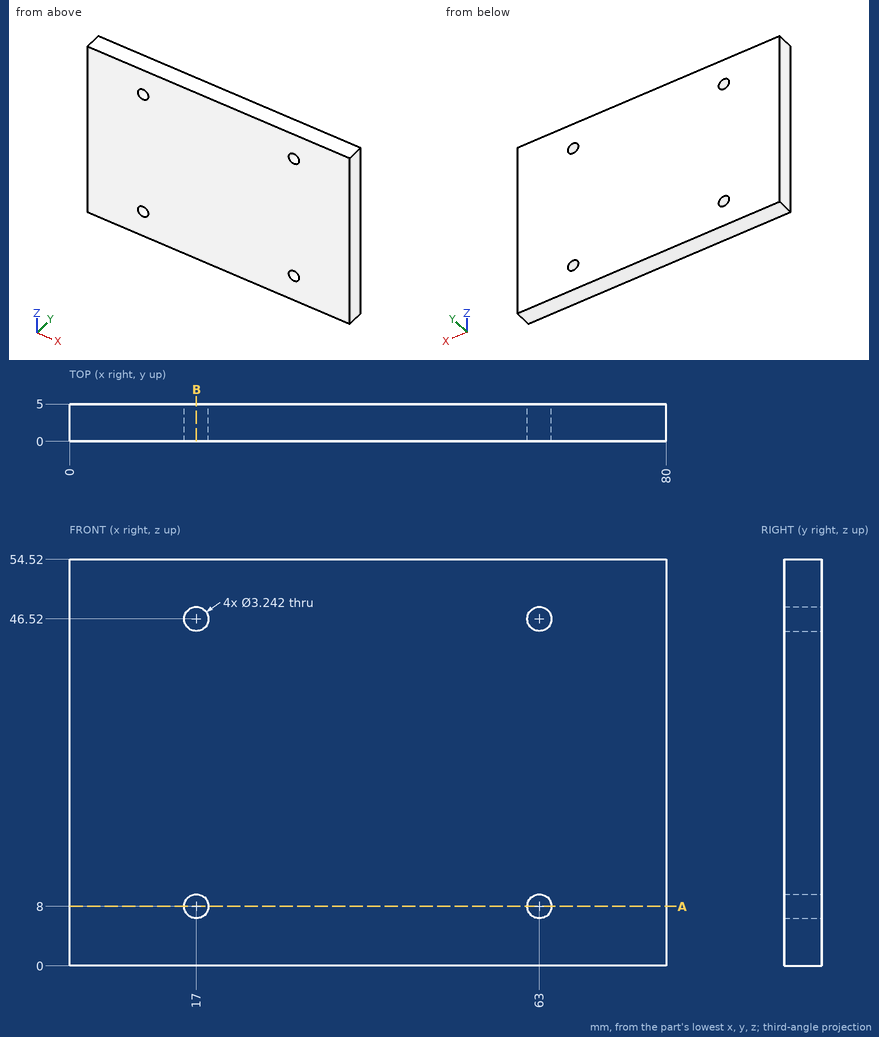
Input: dimensioned drawing with shaded views. Units: mm. Origin: part minimum x, y, z. Round coordinates to 2 decimals unless told otherwise and drop trailing zeros. Order: outer loops, then holes, each group sorted by start corner. A loop starts at its lowest first (then second) coordinate and runs counter-clockwise, first axis right, second up. Notation, with made-up numbers: M -40,66 L -27,66 A20 ccw -27,89 Z; hole C -22,7.25 d4. An arc over 180 degrees is marked long. Use one line per item in the form item = value. Start each with the question number.
Q1. Material intervals for line 1 (X direction, y = 3.5, z = 46.52); line 2 (Z direction, x = 63, y = 2.6); line 3 (X direction, y = 1, z = 9), sorted ascending. Write a range as [from, to].
Q2. Cut plane A-A (z = 8). Return loops of the section in (x, y), and give its area (3 significant figures).
Q3. Cut plane B-B (x = 17). Return loops of the section in (y, z), and give its area (3 significant figures).
Q4. Pin query (flat end, axial travel): pin 1 Ø3 at (x, z) = (17, 8) entering from -Y. Return the tip coordinate at first contact, or that it passes through.
Geometry results:
q1.line_1 = [0, 15.38], [18.62, 61.38], [64.62, 80]
q1.line_2 = [0, 6.38], [9.62, 44.9], [48.14, 54.52]
q1.line_3 = [0, 15.72], [18.28, 61.72], [64.28, 80]
q2.outline = M 0,0 L 15.38,0 L 15.38,5 L 0,5 Z; M 18.62,0 L 61.38,0 L 61.38,5 L 18.62,5 Z; M 64.62,0 L 80,0 L 80,5 L 64.62,5 Z
q2.area = 368 mm^2
q3.outline = M 0,0 L 5,0 L 5,6.38 L 0,6.38 Z; M 0,9.62 L 5,9.62 L 5,44.9 L 0,44.9 Z; M 0,48.14 L 5,48.14 L 5,54.52 L 0,54.52 Z
q3.area = 240 mm^2
q4.pin_1 = through
